Source: three-view drawing plus pictorial views. Frame: mm from the lowest corner of the part. A direction names the side the tool comes from. Coordinates: 2 decimals unless noted, no trailing zeros. Write each loop counter-clockwise with the first axis right and the second up, starting at its lowest first coordinate (ties: lowest second). Pieces come first, ordered by that corner, then holes. Notation, with made-up numbers: (73, 0.25) - (94, 0.25) arc R29 cw to (94, 39.25) - close; hole circle Ø1 at (21, -18). An arc over 180 degrees is marked (long way). Put each result on its own line as item: value. Start each with the question number.
1. Pin query (flat end, axial travel): pin 1 (6 mm diameter, centred on x = 10, z = 12, fed in from +Y); pin 2 (3.5 mm diameter, centred on x = 8, y = 6, fed in from -Z); pin 3 (5 mm diameter, centred on y = 7.5, z = 11.5, fed in from +X). Return the tip coordinate at first contact, or that it passes through.
2. Line query: line 1 (Y direction, x = 0.2, z = 8); line 2 (X direction, y = 19.5, z = 11); line 3 (Z direction, x = 5, y = 12). Output: solid intervals per line, ascending.
3. Access query for the marked faces 1 and 2. Directions: +Z, -Z, +X, -X, +Y, -Y. A direction counts if a zero-diameter tool reaches every point of the face in a straight line with its end or side. Return the directions, or none.
4. Cut plane B-B, the plane z = 8. Return loops of the section in (x, y).
5. Cut plane A-A, the plane x = 8. Return loops of the section in (y, z), and give its area (3 significant figures).
6. Cut plane D-D, the plane y = 13.5. Return loops of the section in (x, z), and give its area (3 significant figures).
7. Cut plane C-C, the plane y = 24. Return loops of the section in (x, z), and give its area (3 significant figures).
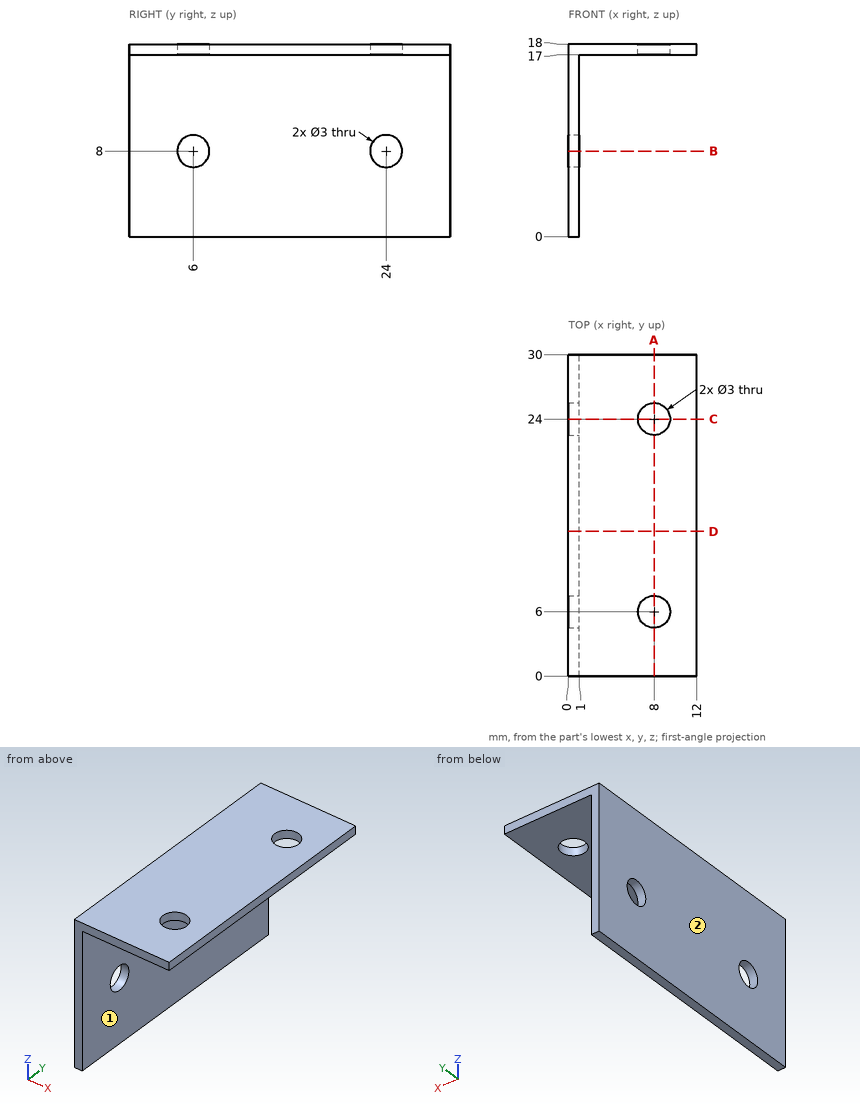
Report:
1. pin 1: passes through
1. pin 2: stops at z = 17
1. pin 3: stops at x = 1
2. line 1: y = 0 to 4.5, 7.5 to 22.5, 25.5 to 30
2. line 2: x = 0 to 1
2. line 3: z = 17 to 18
3. face 1: -Z, +X, +Y, -Y
3. face 2: +Z, -Z, -X, +Y, -Y
4. outline: (0, 0) - (1, 0) - (1, 4.5) - (0, 4.5) - close; (0, 7.5) - (1, 7.5) - (1, 22.5) - (0, 22.5) - close; (0, 25.5) - (1, 25.5) - (1, 30) - (0, 30) - close
5. outline: (0, 17) - (4.5, 17) - (4.5, 18) - (0, 18) - close; (7.5, 17) - (22.5, 17) - (22.5, 18) - (7.5, 18) - close; (25.5, 17) - (30, 17) - (30, 18) - (25.5, 18) - close
5. area: 24.0 mm^2
6. outline: (0, 0) - (1, 0) - (1, 17) - (12, 17) - (12, 18) - (0, 18) - close
6. area: 29.0 mm^2
7. outline: (0, 0) - (1, 0) - (1, 6.5) - (0, 6.5) - close; (0, 9.5) - (1, 9.5) - (1, 17) - (6.5, 17) - (6.5, 18) - (0, 18) - close; (9.5, 17) - (12, 17) - (12, 18) - (9.5, 18) - close
7. area: 23.0 mm^2
